Build history of the part. All positions in model axes, mm. A direction names the side the tool comes from. Coordinates: 2 decimals unless noted, no trailing zeros. Write each loop counter-clockwise with the first axis right and the second up, starting at its lowest first coordinate (ties: lowest second). Pieces come first, ordered by that corner, then holes.
```python
from build123d import *

# Parameters (mm, degrees)
SKETCH_W                     = 110
SKETCH_H                     = 84
PAD_DEPTH                    = 5
SKETCH001_R                  = 1.45
HOLE_DEPTH                   = 281.991975
POCKET_DEPTH                 = 1.75
SKETCH001_LINEARPATTERN_2_R  = 1.45
HOLE_LINEARPATTERN_2_DEPTH   = 281.991975
POCKET_LINEARPATTERN_2_DEPTH = 1.75
LINEARPATTERN001_COUNT       = 2
LINEARPATTERN001_PITCH       = 58
MULTITRANSFORM_FACE2_W       = 84
MULTITRANSFORM_FACE2_H       = 5
PAD001_DEPTH                 = 17
PAD001_FACE6_W               = 84
PAD001_FACE6_H               = 17
PAD002_DEPTH                 = 5
POCKET001_DEPTH              = 315.189466
POCKET002_DEPTH              = 10.001
FILLET_R                     = 5
FILLET001_R                  = 4


with BuildPart() as part:
    # Sketch → Pad (new body)
    with BuildSketch(Plane.XY):
        Rectangle(SKETCH_W, SKETCH_H)
    extrude(amount=PAD_DEPTH)

    # Sketch001 (on Face6 of Pad) → Hole (cut, through all)
    with BuildSketch(Plane.XY.offset(5)):
        with Locations((-46, 33)):
            Circle(SKETCH001_R)
    hole = extrude(amount=-HOLE_DEPTH, mode=Mode.SUBTRACT)

    # Sketch002 (on Face4 of Hole) → Pocket (cut)
    with BuildSketch(Plane(origin=(0, 0, 0), x_dir=(1, 0, 0), z_dir=(0, 0, -1))):
        Polygon((-46, -36.031089), (-43.375, -34.515544), (-43.375, -31.484456), (-46, -29.968911), (-48.625, -31.484456), (-48.625, -34.515544), align=None)
    pocket = extrude(amount=-POCKET_DEPTH, mode=Mode.SUBTRACT)

    # Sketch001 LinearPattern 2 → Hole LinearPattern 2 (cut, through all)
    with BuildSketch(Plane(origin=(86, 0, 5), x_dir=(1, 0, 0), z_dir=(0, 0, 1))):
        with Locations((-46, 33)):
            Circle(SKETCH001_LINEARPATTERN_2_R)
    hole_linearpattern_2 = extrude(amount=-HOLE_LINEARPATTERN_2_DEPTH, mode=Mode.SUBTRACT)

    # Sketch002 LinearPattern 2 → Pocket LinearPattern 2 (cut)
    with BuildSketch(Plane(origin=(86, 0, 0), x_dir=(1, 0, 0), z_dir=(0, 0, -1))):
        Polygon((-46, -36.031089), (-43.375, -34.515544), (-43.375, -31.484456), (-46, -29.968911), (-48.625, -31.484456), (-48.625, -34.515544), align=None)
    pocket_linearpattern_2 = extrude(amount=-POCKET_LINEARPATTERN_2_DEPTH, mode=Mode.SUBTRACT)

    # LinearPattern001: Hole, Pocket, Hole LinearPattern 2, Pocket LinearPattern 2 ×2
    with Locations(*[(0, -i * LINEARPATTERN001_PITCH, 0) for i in range(1, LINEARPATTERN001_COUNT)]):
        add(hole, mode=Mode.SUBTRACT)
        add(pocket, mode=Mode.SUBTRACT)
        add(hole_linearpattern_2, mode=Mode.SUBTRACT)
        add(pocket_linearpattern_2, mode=Mode.SUBTRACT)

    # MultiTransform Face2 → Pad001 (add)
    with BuildSketch(Plane(origin=(-55, 0, 2.5), x_dir=(0, 1, 0), z_dir=(-1, 0, 0))):
        Rectangle(MULTITRANSFORM_FACE2_W, MULTITRANSFORM_FACE2_H)
    pad001 = extrude(amount=PAD001_DEPTH)

    # Pad001 Face6 → Pad002 (add)
    with BuildSketch(Plane(origin=(-63.5, 0, 0), x_dir=(0, -1, 0), z_dir=(0, 0, -1))):
        Rectangle(PAD001_FACE6_W, PAD001_FACE6_H)
    pad002 = extrude(amount=PAD002_DEPTH)

    # Sketch003 (on Face7 of Pad002) → Pocket001 (cut, through all)
    with BuildSketch(Plane.XY.offset(5)):
        with BuildLine():
            ThreePointArc((-59.95, 32.5), (-63.5, 36.05), (-67.05, 32.5))
            Line((-67.05, 32.5), (-67.05, -32.5))
            ThreePointArc((-67.05, -32.5), (-63.5, -36.05), (-59.95, -32.5))
            Line((-59.95, 32.5), (-59.95, -32.5))
        make_face()
    pocket001 = extrude(amount=-POCKET001_DEPTH, mode=Mode.SUBTRACT)

    # Mirrored: Pad001, Pad002, Pocket001 across YZ
    add(pad001.mirror(Plane.YZ))
    add(pad002.mirror(Plane.YZ))
    add(pocket001.mirror(Plane.YZ), mode=Mode.SUBTRACT)

    # Sketch004 (on Face5 of Mirrored) → Pocket002 (cut, through all)
    with BuildSketch(Plane.XY.offset(5)):
        Polygon((-38.540481, 34), (32.540481, 34), (-3, 10.030838), align=None)
        Polygon((-51.95, -22.981952), (-51.95, 30.981952), (-11.942278, 4), align=None)
        Polygon((-50.40255, -34), (44.40255, -34), (-3, -2.030838), align=None)
        Polygon((51.95, 35.028464), (51.95, -27.028464), (5.942278, 4), align=None)
    extrude(amount=-POCKET002_DEPTH, mode=Mode.SUBTRACT)

    # Fillet
    fillet_edges = [part.edges().sort_by_distance(p)[0] for p in [
        (-51.95, 30.981952, 2.5),
        (-51.95, -22.981952, 2.5),
        (-11.942278, 4, 2.5),
        (44.40255, -34, 2.5),
        (-50.40255, -34, 2.5),
        (-3, -2.030838, 2.5),
        (5.942278, 4, 2.5),
        (51.95, -27.028464, 2.5),
        (51.95, 35.028464, 2.5),
        (-38.540481, 34, 2.5),
        (-3, 10.030838, 2.5),
        (32.540481, 34, 2.5),
    ]]
    fillet(fillet_edges, radius=FILLET_R)

    # Fillet001
    fillet001_edges = [part.edges().sort_by_distance(p)[0] for p in [
        (-72, 42, 2.5),
        (-72, 42, -2.5),
        (-72, -42, -2.5),
        (-72, -42, 2.5),
        (72, 42, 2.5),
        (72, 42, -2.5),
        (72, -42, 2.5),
        (72, -42, -2.5),
        (55, 42, -2.5),
        (55, -42, -2.5),
        (-55, 42, -2.5),
        (-55, -42, -2.5),
    ]]
    fillet(fillet001_edges, radius=FILLET001_R)


solid = part.part
```
1. Mould opens along Y. For faces 1 (the face through (-1, 42, 1)), 2 (the face through (-67.05, 0, 0)), 3 (the face through (-47.15, -25.88, 3.4)), 4 (the face through (56.203, -40.859, -2.535)) say: +Y half, -Y half, draft (parallel to the pull), parting line (faces both ways), or undercut.
Computed values:
face 1: +Y half
face 2: undercut
face 3: undercut
face 4: -Y half
2. Saw through at C-C on x = 3.5. List the corners of the cut face in (y, z), plus the area to 3 significant figures.
Computed values:
outline: (-42, 0) - (-34, 0) - (-34, 5) - (-42, 5) - close; (-6.41, 0) - (14.41, 0) - (14.41, 5) - (-6.41, 5) - close; (34, 0) - (42, 0) - (42, 5) - (34, 5) - close
area: 184 mm2
3. Saw through at A-A on z = -2.75. List the corners of the cut face in (x, y).
Computed values:
outline: (-72, -38) arc R4 ccw to (-68, -42) - (-59, -42) arc R4 ccw to (-55, -38) - (-55, 38) arc R4 ccw to (-59, 42) - (-68, 42) arc R4 ccw to (-72, 38) - close; (55, -38) arc R4 ccw to (59, -42) - (68, -42) arc R4 ccw to (72, -38) - (72, 38) arc R4 ccw to (68, 42) - (59, 42) arc R4 ccw to (55, 38) - close; hole (-67.05, -32.5) arc R3.55 ccw to (-59.95, -32.5) - (-59.95, 32.5) arc R3.55 ccw to (-67.05, 32.5) - close; hole (59.95, -32.5) arc R3.55 ccw to (67.05, -32.5) - (67.05, 32.5) arc R3.55 ccw to (59.95, 32.5) - close
4. Saw through at D-D on y = -7.5. List the corners of the cut face in (x, z).
Computed values:
outline: (-72, -5) - (-67.05, -5) - (-67.05, 5) - (-72, 5) - close; (-59.95, -5) - (-55, -5) - (-55, 0) - (-51.95, 0) - (-51.95, 5) - (-59.95, 5) - close; (-28.99, 0) - (-11.11, 0) - (-11.11, 5) - (-28.99, 5) - close; (5.11, 0) - (22.99, 0) - (22.99, 5) - (5.11, 5) - close; (51.95, 0) - (55, 0) - (55, -5) - (59.95, -5) - (59.95, 5) - (51.95, 5) - close; (67.05, -5) - (72, -5) - (72, 5) - (67.05, 5) - close
5. Flat gauge pins, fed straight in: pin 1 (4 mm diameter, centred on x = 40.5, y = 32.5, fed in from -Z); pin 2 (4 mm diameter, centred on x = -46, y = 33, fed in from +Z). Where does each tip first touch, or does it go through?
Computed values:
pin 1: stops at z = 0
pin 2: stops at z = 5
6. 3-axis set-ups, long thin cutter, end or side, ignore diameter. For faces 5 (the face through (-56.203, -40.859, -2.535)), 6 (the face through (-56.203, 40.859, -2.535)), 7 (the face through (41.1, -23.7, 1.75)), 8 (the face through (32.8, -30.55, 2.46)): which of +Z, -Z, +X, -X, +Y, -Y reach the whole face in a straight line?
Computed values:
face 5: -Z, -Y
face 6: -Z, +Y
face 7: -Z
face 8: +Z, -Z
7. Probe line 1 along X through (y, z) = (4.5, 2.25); line 2 along X through (y, z) = (-26, -4). List the from-to ranges inside material, lowest first.
Computed values:
line 1: x = -72 to -67.05, -59.95 to -51.95, -15.91 to 9.91, 51.95 to 59.95, 67.05 to 72
line 2: x = -72 to -67.05, -59.95 to -55, 55 to 59.95, 67.05 to 72
8. Saw through at B-B on x = 63.5. List the corners of the cut face in (y, z), plus the area to 3 significant figures.
Computed values:
outline: (-42, -5) - (-36.05, -5) - (-36.05, 5) - (-42, 5) - close; (36.05, -5) - (42, -5) - (42, 5) - (36.05, 5) - close
area: 119 mm2
